Part model, mm, in its own coordinate system. Face numbers are marked on the shaded views. A direction names the side the tool comes from. Coordinates: 2 decimals unless noted, no trailing zeros. Write each loop counter-clockwise with the first axis right and the second up, starting at its lowest first coordinate (ties: lowest second). Pieces come first, ordered by that corner, then holes. Notation, with made-up numbers: M 57.25,-31 L 109.25,-31 A15 cw 109.25,-8 Z; hole C 68.25,42.25 d9. An arc over 180 degrees is marked long. Use a Markdown table: item, result. Add a question column.
Q1. Wall check: L1, parallel to Y at x = 27.5, z = 4.25; L2, parallel to X at y = -13.5, z = 15.25; L3, parallel to Z at x = -3, y = 18. Give the ranges that are in metal, low to high. Write a range as from..to.
Q2. Mould opens along Y. For the marked faces 3, 4 and 5 say: released by +Y, released by -Y, zero draft, split by the parting line, or undercut.
Q3. Slice it at A-A on x = -15. Write the cut outline in (y, z), then the cut area to 3 significant figures.
Q4. Slice it at D-D on z = 16.25. Write the cut outline in (x, y), then the cut area to 3 significant figures.
Q5. Tool access for the marked faces 1 and 2: list every direction of +Z, -Z, +X, -X, +Y, -Y with a clear straight run to the whole face (end or side of a thin tool).
Q6. Slice it at C-C on x = 12. Write the cut outline in (y, z), then the cut area to 3 significant figures.
Q7. Pin check, flat tips, straight feed: pin 1 Ø5 at (x, y) = (21.5, -10.5) entering from +Z; pin 2 Ø2 at (x, y) = (-5.5, 25.5) entering from +Z. Stop position of each tip, or through.
Q8. Slice it at B-B on z = 22.25. Write the cut outline in (x, y), then the cut area to 3 significant figures.
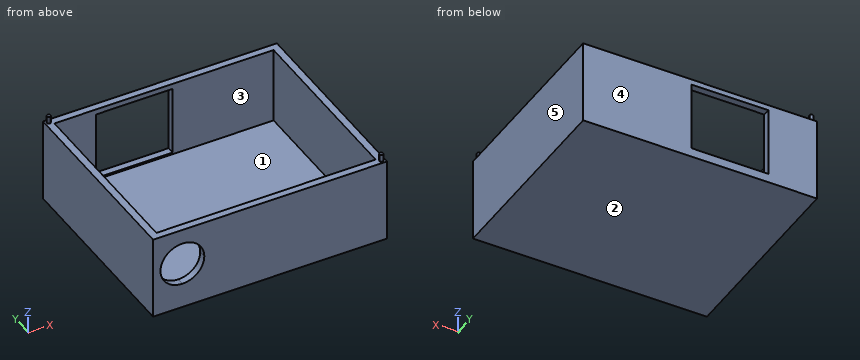
from build123d import *

# Parameters (mm, degrees)
F0_W          = 64
F0_H          = 54
F1_DEPTH      = 23
F2_W          = 60
F2_H          = 50
F3_DEPTH      = 21
F5_DEPTH      = 25.4
F5_DEPTH_BACK = 25.4
F7_DEPTH      = 25.4
F7_DEPTH_BACK = 25.4
F11_DEPTH     = 2
F13_DEPTH     = 2


with BuildPart() as f1:
    # F0 (on Top) → F1 (new body)
    with BuildSketch(Plane.XY):
        Rectangle(F0_W, F0_H)
    extrude(amount=F1_DEPTH)

    # F2 (on face) → F3 (cut)
    with BuildSketch(Plane.XY.offset(23)):
        Rectangle(F2_W, F2_H)
    extrude(amount=-F3_DEPTH, mode=Mode.SUBTRACT)

    # F4 (on face) → F5 (cut, two sides)
    with BuildSketch(Plane(origin=(0, -25, 0), x_dir=(-1, 0, 0), z_dir=(0, 1, 0))) as f5_sk:
        with BuildLine():
            ThreePointArc((24, 6.93), (28.2426406871, 8.6873593129), (30, 12.93))
            ThreePointArc((30, 12.93), (28.2426406871, 17.1726406871), (24, 18.93))
            ThreePointArc((24, 18.93), (19.7573593129, 17.1726406871), (18, 12.93))
            ThreePointArc((18, 12.93), (19.7573593129, 8.6873593129), (24, 6.93))
        make_face()
    extrude(amount=-F5_DEPTH, mode=Mode.SUBTRACT)
    extrude(f5_sk.sketch, amount=F5_DEPTH_BACK, mode=Mode.SUBTRACT)

    # F6 (on face) → F7 (cut, two sides)
    with BuildSketch(Plane.XZ.offset(-25)) as f7_sk:
        Polygon((-18.6692412496, 2.5), (-8.1692412496, 2.5), (2.3307587504, 2.5), (2.3307587504, 21.5), (-18.6692412496, 21.5), align=None)
    extrude(amount=-F7_DEPTH, mode=Mode.SUBTRACT)
    extrude(f7_sk.sketch, amount=F7_DEPTH_BACK, mode=Mode.SUBTRACT)

    # F10 (on face) → F11 (join)
    with BuildSketch(Plane.XY.offset(23)):
        with BuildLine():
            Line((-30.6464466094, 26.3535533906), (-31, 26))
            Line((-31, 26), (-30.6464466094, 25.6464466094))
            ThreePointArc((-30.6464466094, 25.6464466094), (-30.5380602337, 25.8086582838), (-30.5, 26))
            ThreePointArc((-30.5, 26), (-30.5380602337, 26.1913417162), (-30.6464466094, 26.3535533906))
        make_face()
        with BuildLine():
            ThreePointArc((-30.6464466094, 26.3535533906), (-31, 26.5), (-31.3535533906, 26.3535533906))
            Line((-31.3535533906, 26.3535533906), (-31, 26))
            Line((-31, 26), (-30.6464466094, 26.3535533906))
        make_face()
        with BuildLine():
            Line((-31, 26), (-31.3535533906, 26.3535533906))
            ThreePointArc((-31.3535533906, 26.3535533906), (-31.5, 26), (-31.3535533906, 25.6464466094))
            Line((-31.3535533906, 25.6464466094), (-31, 26))
        make_face()
        with BuildLine():
            Line((-30.6464466094, 25.6464466094), (-31, 26))
            Line((-31, 26), (-31.3535533906, 25.6464466094))
            ThreePointArc((-31.3535533906, 25.6464466094), (-31, 25.5), (-30.6464466094, 25.6464466094))
        make_face()
    extrude(amount=F11_DEPTH)

    # F12 (on face) → F13 (join)
    with BuildSketch(Plane.XY.offset(23)):
        with BuildLine():
            Line((31, -26), (30.6464466094, -25.6464466094))
            ThreePointArc((30.6464466094, -25.6464466094), (30.5, -26), (30.6464466094, -26.3535533906))
            Line((30.6464466094, -26.3535533906), (31, -26))
        make_face()
        with BuildLine():
            ThreePointArc((31.3535533906, -25.6464466094), (31, -25.5), (30.6464466094, -25.6464466094))
            Line((30.6464466094, -25.6464466094), (31, -26))
            Line((31, -26), (31.3535533906, -25.6464466094))
        make_face()
        with BuildLine():
            Line((31.3535533906, -25.6464466094), (31, -26))
            Line((31, -26), (31.3535533906, -26.3535533906))
            ThreePointArc((31.3535533906, -26.3535533906), (31.4619397663, -26.1913417162), (31.5, -26))
            ThreePointArc((31.5, -26), (31.4619397663, -25.8086582838), (31.3535533906, -25.6464466094))
        make_face()
        with BuildLine():
            Line((31.3535533906, -26.3535533906), (31, -26))
            Line((31, -26), (30.6464466094, -26.3535533906))
            ThreePointArc((30.6464466094, -26.3535533906), (31, -26.5), (31.3535533906, -26.3535533906))
        make_face()
    extrude(amount=F13_DEPTH)


solid = f1.part
Recorded:
| question | item | result |
|---|---|---|
| 1 | L1 | -27..-25, 25..27 |
| 1 | L2 | -32..-30, 30..32 |
| 1 | L3 | 0..2 |
| 2 | face 3 | undercut |
| 2 | face 4 | released by +Y |
| 2 | face 5 | zero draft |
| 3 | outline | M -27,0 L 27,0 L 27,2.5 L 25,2.5 L 25,2 L -25,2 L -25,23 L -27,23 Z; M 25,21.5 L 27,21.5 L 27,23 L 25,23 Z |
| 3 | area | 154 mm² |
| 4 | outline | M -32,-27 L -29,-27 L -29,-25 L -30,-25 L -30,25 L -18.67,25 L -18.67,27 L -32,27 Z; M -19,-27 L 32,-27 L 32,27 L 2.33,27 L 2.33,25 L 30,25 L 30,-25 L -19,-25 Z |
| 4 | area | 394 mm² |
| 5 | face 1 | +Z |
| 5 | face 2 | -Z, +X, -X, +Y, -Y |
| 6 | outline | M -27,0 L 27,0 L 27,23 L 25,23 L 25,2 L -25,2 L -25,23 L -27,23 Z |
| 6 | area | 192 mm² |
| 7 | pin 1 | z = 2 |
| 7 | pin 2 | z = 23 |
| 8 | outline | M -32,-27 L 32,-27 L 32,27 L -32,27 Z; hole M -30,-25 L 30,-25 L 30,25 L -30,25 Z |
| 8 | area | 456 mm² |
